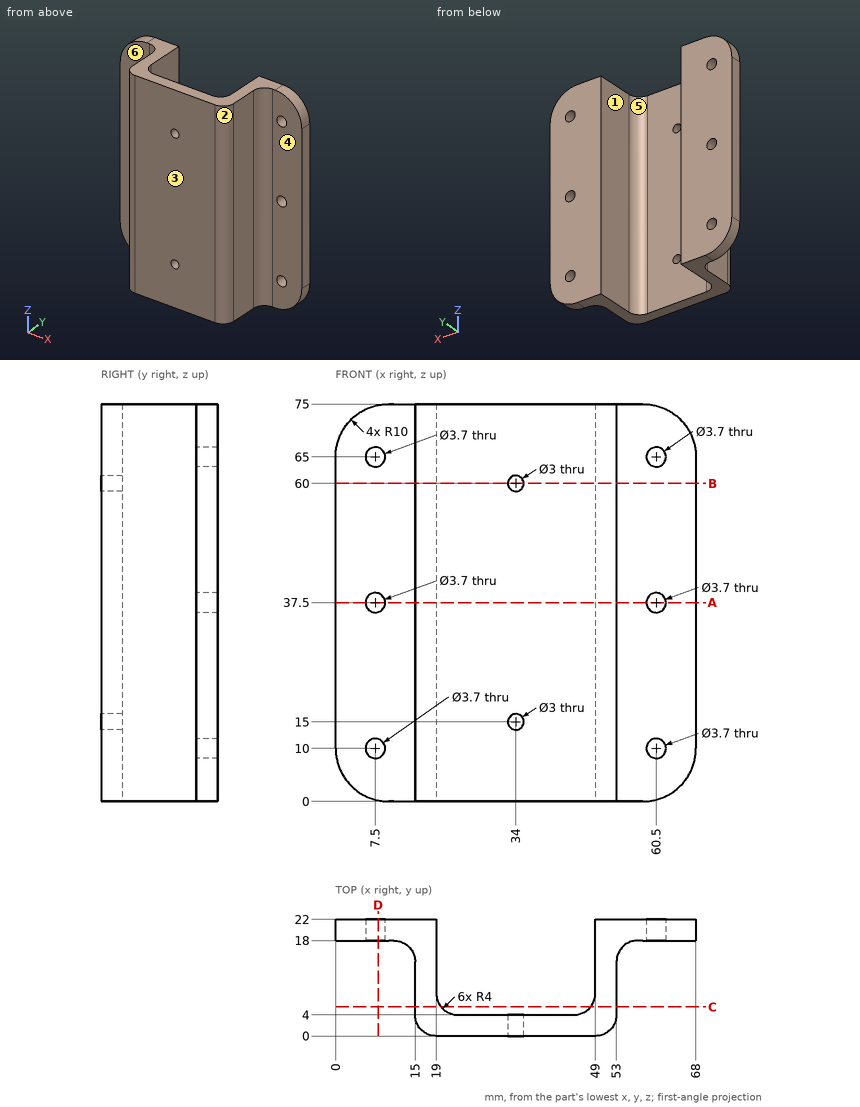
Job drawing, mm, ordinate dimensions from the low corner. One solid piece. A direction names the side the tool comes from. Round coordinates to 2 decimals unless told otherwise and drop trailing zeros. Loops run counter-clockwise (first coordinate to the right, second up) from the corner with the lowest first, then second, coordinate; pieces in that order, holes last. Notation, with made-up numbers: M 24.5,83 L 83.5,83 A15 cw 83.5,90 Z; hole C 43,80.5 d3. An arc over 180 degrees is marked long. Answer as CSV lines item,"result".
1. Cut at B-B on z = 60. Write the cut outline in (x, y), then the cut area to 3 significant figures.
Resolved:
outline,"M 0,18 L 11,18 A4 cw 15,14 L 15,4 A4 ccw 19,0 L 32.5,0 L 32.5,4 L 23,4 A4 cw 19,8 L 19,22 L 0,22 Z; M 35.5,0 L 49,0 A4 ccw 53,4 L 53,14 A4 cw 57,18 L 68,18 L 68,22 L 49,22 L 49,8 A4 cw 45,4 L 35.5,4 Z"
area,"411 mm²"
2. Two-plate mould, pull along X, no slides. Class the marked faces 1, 2 and 3: released by +X, released by -X, zero draft, split by the parting line, or undercut.
Resolved:
face 1,"undercut"
face 2,"released by +X"
face 3,"zero draft"
3. Cut at A-A on z = 37.5. Write the cut outline in (x, y), then the cut area to 3 significant figures.
Resolved:
outline,"M 0,18 L 5.65,18 L 5.65,22 L 0,22 Z; M 9.35,18 L 11,18 A4 cw 15,14 L 15,4 A4 ccw 19,0 L 49,0 A4 ccw 53,4 L 53,14 A4 cw 57,18 L 58.65,18 L 58.65,22 L 49,22 L 49,8 A4 cw 45,4 L 23,4 A4 cw 19,8 L 19,22 L 9.35,22 Z; M 62.35,18 L 68,18 L 68,22 L 62.35,22 Z"
area,"393 mm²"
4. 3-axis set-ups, long thin cutter, end or side, ignore diameter. For the marked faces 4, 5 and 6: which of +Z, -Z, +X, -X, +Y, -Y reach the whole face in a straight line?
Resolved:
face 4,"+Z, -Z, +X, -Y"
face 5,"+Z, -Z, +Y"
face 6,"+Z, -Z, -X, -Y"
5. Flat gauge pins, fed straight in: P1, Ø3.5, axis at x = 62.5, z = 29, coming from the -Y side; P2, Ø4, axis at y = 12, z = 49.5, coming from the -X side; P3, Ø24, axis at x = 34, z = 27, coming from the +Y side. Where does each tip first touch, or does it go through?
Resolved:
P1,"stops at y = 18"
P2,"stops at x = 15"
P3,"stops at y = 4.13"
6. Cut at D-D on x = 8. Write the cut outline in (y, z), then the cut area to 3 significant figures.
Resolved:
outline,"M 18,0.2 L 22,0.2 L 22,8.22 L 18,8.22 Z; M 18,11.78 L 22,11.78 L 22,35.72 L 18,35.72 Z; M 18,39.28 L 22,39.28 L 22,63.22 L 18,63.22 Z; M 18,66.78 L 22,66.78 L 22,74.8 L 18,74.8 Z"
area,"256 mm²"
7. Cut at C-C on y = 5.5. Write the cut outline in (x, z).
Resolved:
outline,"M 15,0 L 19.88,0 L 19.88,75 L 15,75 Z; M 48.12,0 L 53,0 L 53,75 L 48.12,75 Z"
8. Wall check: probe 1 along Z at (x, y) = (34, 1.1); probe 2 along X at (y, z) = (8, 9); probe 3 along Z at (x, y) = (7.5, 19.2). Give the ranges that are in metal, low to high. Write a range as [from, to].
Resolved:
probe 1,"z = [0, 13.5], [16.5, 58.5], [61.5, 75]"
probe 2,"x = [15, 19], [49, 53]"
probe 3,"z = [0.32, 8.15], [11.85, 35.65], [39.35, 63.15], [66.85, 74.68]"
